The listing builds one solid part. Answer for the finished solid, in the listing's coordinates (mm). Give positions to 0.01 mm unless a question says otherwise; leave off trailing zeros. Loops run counter-clockwise (first coordinate to the right, second up) from the corner with the lowest first, then second, coordinate; pieces in that order, holes last.
Item 1: Section C-C, the plane y = -1.5 is taken. Give the number of separate pieces and of enclosed holes in the cut face, and give its area (3 significant figures).
Item 2: Section D-D, the plane x = 222.25 is taken. Give the vertices of the cut face in (y, z) (3 decimals), and give its area (3 significant figures).
Item 3: Consider line 1 along X through (y, z) = (-1.5, 143.5); line 2 along Z through (x, y) = (-127, 0.5) (3 decimals); line 3 along Z through (x, y) = (-222.25, -1) (1 decimal). Determine where each line is inside the solid, lowest interval first.
Item 4: Section B-B, the plane z = -144 is taken. Give the vertices of the cut face in (x, y) (1 decimal), and give its area (3 significant figures).
Item 5: Each of these flat-tipped pins is pushed along its axis until it touches: pin 1 Ø3 at (x, z) = (-185.47, 106.65) entering from +Y; pin 2 Ø3 at (x, y) = (10.5, 0) entering from +Z (3 decimals); pin 3 Ø1.5 at (y, z) = (1.5, 51) entering from +X; pin 4 Ø3 at (y, z) = (0.5, 132) entering from +X. Where does it stop, or does it pass through?
Item 6: The mould has two halves that part along Z. Classify faces 1 (the face through (-4, -3.175, -2)), 2 (the face through (202.324, -0.044, 74.911)), 3 (the face through (220.39, 0.04, -150.13)): pulls with the +Z half, pulls with the -Z half, needs draft (parallel to the pull), parting line crosses it, or undercut.
Item 7: Section A-A, the plane x = 127 is taken. Give the vertices of the cut face in (y, z) (3 decimals), and give its area (3 significant figures).
from build123d import *

# Parameters (mm, degrees)
SKETCH1_W               = 504.825
SKETCH1_H               = 336.55
BOSS_EXTRUDE1_DEPTH     = 3.175
SKETCH2_R               = 14.2748
CUT_EXTRUDE1_DEPTH      = 7.35
CUT_EXTRUDE3_DEPTH      = 7.35
SKETCH6_W               = 114.3
SKETCH6_H               = 76.2
CUT_EXTRUDE4_DEPTH      = 7.35
SKETCH8_R               = 2.413
SKETCH8_R_2             = 9.525
BOSS_EXTRUDE3_DEPTH     = 3.175
CUT_EXTRUDE5_DEPTH      = 4.175
CUT_EXTRUDE5_DEPTH_BACK = 4.175


with BuildPart() as part:
    # Sketch1 → Boss-Extrude1 (new body, symmetric)
    with BuildSketch(Plane(origin=(0, 0, 0), x_dir=(1, 0, 0), z_dir=(0, 1, 0))):
        Rectangle(SKETCH1_W, SKETCH1_H)
    extrude(amount=BOSS_EXTRUDE1_DEPTH, both=True)

    # Sketch2 → Cut-Extrude1 (cut, through all)
    with BuildSketch(Plane(origin=(0, 3.175, 0), x_dir=(1, 0, 0), z_dir=(0, 1, 0))):
        with Locations((-222.25, 135.975286336)):
            Circle(SKETCH2_R)
        with Locations((222.25, 135.975286336)):
            Circle(SKETCH2_R)
        with Locations((-127, -124.374713664)):
            Circle(SKETCH2_R)
        with Locations((127, -124.374713664)):
            Circle(SKETCH2_R)
    extrude(amount=-CUT_EXTRUDE1_DEPTH, mode=Mode.SUBTRACT)

    # Sketch5 → Cut-Extrude3 (cut, through all)
    with BuildSketch(Plane.XZ.offset(3.175)):
        Polygon((252.4125, 168.275), (252.4125, -15.875), (150.8125, 168.275), align=None)
        Polygon((-252.4125, -15.875), (-150.8125, 168.275), (-252.4125, 168.275), align=None)
    extrude(amount=-CUT_EXTRUDE3_DEPTH, mode=Mode.SUBTRACT)

    # Sketch6 → Cut-Extrude4 (cut, through all)
    with BuildSketch(Plane(origin=(0, 3.175, 0), x_dir=(1, 0, 0), z_dir=(0, 1, 0))):
        with Locations((0, -130.175)):
            Rectangle(SKETCH6_W, SKETCH6_H)
    extrude(amount=-CUT_EXTRUDE4_DEPTH, mode=Mode.SUBTRACT)

    # Sketch8 → Boss-Extrude3 (add, symmetric)
    with BuildSketch(Plane(origin=(0, 0, 0), x_dir=(1, 0, 0), z_dir=(0, 1, 0))):
        with Locations((-185.4708, -106.645513664)):
            Circle(SKETCH8_R)
        Polygon((-252.4125, 15.875), (-150.8125, -168.275), (-252.4125, -168.275), align=None)
        with Locations((-220.9292, -142.103913664)):
            Circle(SKETCH8_R, mode=Mode.SUBTRACT)
        with Locations((-203.2, -124.374713664)):
            Circle(SKETCH8_R_2, mode=Mode.SUBTRACT)
        with BuildLine():
            ThreePointArc((-183.0578, -106.645513664), (-184.003859621, -104.729618332), (-186.100199439, -104.316044767))
            Line((-186.100199439, -104.316044767), (-183.83584242, -108.420191864))
            ThreePointArc((-183.83584242, -108.420191864), (-183.260854114, -107.614383201), (-183.0578, -106.645513664))
        make_face()
        with BuildLine():
            Line((-183.83584242, -108.420191864), (-186.100199439, -104.316044767))
            ThreePointArc((-186.100199439, -104.316044767), (-187.583568952, -107.811179293), (-183.83584242, -108.420191864))
        make_face()
    extrude(amount=BOSS_EXTRUDE3_DEPTH, both=True)

    # Sketch8<3> → Cut-Extrude5 (cut, two sides)
    with BuildSketch(Plane(origin=(0, 0, 0), x_dir=(1, 0, 0), z_dir=(0, 1, 0))) as cut_extrude5_sk:
        with BuildLine():
            ThreePointArc((-183.0578, -106.645513664), (-184.003859621, -104.729618332), (-186.100199439, -104.316044767))
            Line((-186.100199439, -104.316044767), (-183.83584242, -108.420191864))
            ThreePointArc((-183.83584242, -108.420191864), (-183.260854114, -107.614383201), (-183.0578, -106.645513664))
        make_face()
        with BuildLine():
            Line((-183.83584242, -108.420191864), (-186.100199439, -104.316044767))
            ThreePointArc((-186.100199439, -104.316044767), (-187.583568952, -107.811179293), (-183.83584242, -108.420191864))
        make_face()
    extrude(amount=CUT_EXTRUDE5_DEPTH, mode=Mode.SUBTRACT)
    extrude(cut_extrude5_sk.sketch, amount=-CUT_EXTRUDE5_DEPTH_BACK, mode=Mode.SUBTRACT)


solid = part.part
Worked answers:
1. separate pieces: 1
1. enclosed holes: 7
1. area: 149,000 mm2
2. outline: (-3.175, -168.275) - (3.175, -168.275) - (3.175, -150.25) - (-3.175, -150.25) - close; (-3.175, -121.7) - (3.175, -121.7) - (3.175, 38.795) - (-3.175, 38.795) - close
2. area: 1,130 mm2
3. line 1: x = -252.41 to -222.9, -218.96 to -57.15, 57.15 to 164.48
3. line 2: z = -168.275 to 110.1, 138.65 to 168.275
3. line 3: z = -168.3 to -150.3, -121.7 to 140.1, 144.1 to 168.3
4. outline: (-252.4, -3.2) - (-234.1, -3.2) - (-234.1, 3.2) - (-252.4, 3.2) - close; (-210.4, -3.2) - (210.4, -3.2) - (210.4, 3.2) - (-210.4, 3.2) - close; (234.1, -3.2) - (252.4, -3.2) - (252.4, 3.2) - (234.1, 3.2) - close
4. area: 2,910 mm2
5. pin 1: passes through
5. pin 2: stops at z = 92.075
5. pin 3: stops at x = 215.93
5. pin 4: stops at x = 171.65
6. face 1: needs draft
6. face 2: pulls with the +Z half
6. face 3: undercut
7. outline: (-3.175, -168.275) - (3.175, -168.275) - (3.175, 110.1) - (-3.175, 110.1) - close; (-3.175, 138.65) - (3.175, 138.65) - (3.175, 168.275) - (-3.175, 168.275) - close
7. area: 1,960 mm2
